CAD build for the part. Positions are in the model's coordinates, mm. Face numbers are marked on the shaded views. A direction names the side the tool comes from. Give positions to 0.01 mm unless a question says otherwise; leave off trailing zeros. Write each loop counter-clockwise with the first axis right and the second up, starting at its lowest first coordinate (ties: lowest second). Pieces come first, ordered by that corner, then holes. Notation, with made-up numbers: (85, -30.5) - (126, -30.5) arc R24 cw to (126, 5.5) - close; hole circle Ø10 at (74.5, 45). An arc over 180 degrees is marked (long way). Answer as a JSON object with one key per item and string values.
from build123d import *

# Parameters (mm, degrees)
BOSS_EXTRU_1_DEPTH           = 12
ESQUISSE10_R                 = 1.6
ENL_V_MAT_EXTRU_6_DEPTH      = 96.463780217
ENL_V_MAT_EXTRU_1_DEPTH      = 96.463780217
ENL_V_MAT_EXTRU_2_DEPTH      = 11
ESQUISSE4_W                  = 6
ESQUISSE4_H                  = 3
ENL_V_MAT_EXTRU_3_DEPTH      = 9.5
ESQUISSE11_R                 = 5.075
ENL_V_MAT_EXTRU_7_DEPTH      = 2
R_P_TITION_CIRCULAIRE1_COUNT = 3
CHANFREIN1_SIZE              = 0.5


with BuildPart() as part:
    # Esquisse1 → Boss.-Extru.1 (new body)
    with BuildSketch(Plane(origin=(0, 0, 0), x_dir=(1, 0, 0), z_dir=(0, 1, 0))):
        Polygon((-62, -35.79571669), (62, -35.79571669), (0, 71.59143338), align=None)
    extrude(amount=BOSS_EXTRU_1_DEPTH)

    # Esquisse10 → Enlèv. mat.-Extru.6 (cut, through all)
    with BuildSketch(Plane(origin=(0, 12, 0), x_dir=(1, 0, 0), z_dir=(0, 1, 0))):
        with Locations(Location((0, 54, 0), (0, 0, 270))):
            Circle(ESQUISSE10_R)
        with Locations(Location((46.765371804, -27, 0), (0, 0, 270))):
            Circle(ESQUISSE10_R)
        with Locations(Location((-46.765371804, -27, 0), (0, 0, 270))):
            Circle(ESQUISSE10_R)
    extrude(amount=-ENL_V_MAT_EXTRU_6_DEPTH, mode=Mode.SUBTRACT)

    # Esquisse2 → Enlèv. mat.-Extru.1 (cut, through all)
    with BuildSketch(Plane(origin=(0, 12, 0), x_dir=(1, 0, 0), z_dir=(0, 1, 0))):
        Polygon((-8.660254038, 56.59143338), (8.660254038, 56.59143338), (0, 71.59143338), align=None)
        Polygon((62, -35.79571669), (53.339745962, -20.79571669), (44.679491924, -35.79571669), align=None)
        Polygon((-62, -35.79571669), (-44.679491924, -35.79571669), (-53.339745962, -20.79571669), align=None)
    extrude(amount=-ENL_V_MAT_EXTRU_1_DEPTH, mode=Mode.SUBTRACT)

    # Esquisse3 → Enlèv. mat.-Extru.2 (cut)
    with BuildSketch(Plane(origin=(0, 12, 0), x_dir=(1, 0, 0), z_dir=(0, 1, 0))):
        with BuildLine():
            Line((44.679491924, -11.79571669), (12.124355653, 44.59143338))
            ThreePointArc((12.124355653, 44.59143338), (0, 51.59143338), (-12.124355653, 44.59143338))
            Line((-12.124355653, 44.59143338), (-44.679491924, -11.79571669))
            ThreePointArc((-44.679491924, -11.79571669), (-44.679491924, -25.79571669), (-32.555136271, -32.79571669))
            Line((-32.555136271, -32.79571669), (32.555136271, -32.79571669))
            ThreePointArc((32.555136271, -32.79571669), (44.679491924, -25.79571669), (44.679491924, -11.79571669))
        make_face()
    extrude(amount=-ENL_V_MAT_EXTRU_2_DEPTH, mode=Mode.SUBTRACT)

    # Esquisse4 → Enlèv. mat.-Extru.3 (cut)
    with BuildSketch(Plane(origin=(0, 12, 0), x_dir=(1, 0, 0), z_dir=(0, 1, 0))):
        Polygon((29.901923789, 13.799782134), (26.901923789, 18.995934556), (29.5, 20.495934556), (32.5, 15.299782134), align=None)
        with Locations((0, -34.29571669)):
            Rectangle(ESQUISSE4_W, ESQUISSE4_H)
        Polygon((-29.5, 20.495934556), (-26.901923789, 18.995934556), (-29.901923789, 13.799782134), (-32.5, 15.299782134), align=None)
    extrude(amount=-ENL_V_MAT_EXTRU_3_DEPTH, mode=Mode.SUBTRACT)

    # Esquisse11 → Enlèv. mat.-Extru.7 (cut)
    with BuildSketch(Plane(origin=(0, 0, 32.79571669), x_dir=(-1, 0, 0), z_dir=(0, 0, -1))):
        with Locations((-17.555136271, 6.5)):
            Circle(ESQUISSE11_R)
        with Locations(Location((17.555136271, 6.5, 0), (0, 0, 180))):
            Circle(ESQUISSE11_R)
    enl_v_mat_extru_7 = extrude(amount=-ENL_V_MAT_EXTRU_7_DEPTH, mode=Mode.SUBTRACT)

    # Répétition circulaire1: Enlèv. mat.-Extru.7 ×3 about axis
    r_p_tition_circulaire1_axis = Axis((0, 0, 0), (0, 1, 0))
    for i in range(1, R_P_TITION_CIRCULAIRE1_COUNT):
        add(enl_v_mat_extru_7.rotate(r_p_tition_circulaire1_axis, i * 360 / R_P_TITION_CIRCULAIRE1_COUNT), mode=Mode.SUBTRACT)

    # Chanfrein1
    # the kernel refuses this chamfer: 0.5 mm, written as the material it takes off along each edge
    with BuildSketch(Plane(origin=(17.555136271, 6.5, 32.79571669), x_dir=(-1, 0, 0), z_dir=(0, -1, 0))) as chanfrein1_piece_1_section:
        Polygon((5.075 + CHANFREIN1_SIZE, 0), (5.075, -CHANFREIN1_SIZE), (5.075, 0), align=None)
    chanfrein1_piece_1 = revolve(axis=Axis((17.555136271, 6.5, 32.79571669), (0, 0, -1)), mode=Mode.PRIVATE)
    chanfrein1_piece_1 = split(chanfrein1_piece_1, bisect_by=Plane(origin=(22.868441697, 1, 33.034022115), z_dir=(0, 1, 0)), keep=Keep.TOP, mode=Mode.PRIVATE)
    add(chanfrein1_piece_1, mode=Mode.SUBTRACT)
    with BuildSketch(Plane(origin=(-17.555136271, 6.5, 32.79571669), x_dir=(1, 0, 0), z_dir=(0, 1, 0))) as chanfrein1_piece_2_section:
        Polygon((5.075 + CHANFREIN1_SIZE, 0), (5.075, -CHANFREIN1_SIZE), (5.075, 0), align=None)
    chanfrein1_piece_2 = revolve(axis=Axis((-17.555136271, 6.5, 32.79571669), (0, 0, -1)), mode=Mode.PRIVATE)
    chanfrein1_piece_2 = split(chanfrein1_piece_2, bisect_by=Plane(origin=(-22.868441724, 1, 33.034022142), z_dir=(0, 1, 0)), keep=Keep.TOP, mode=Mode.PRIVATE)
    add(chanfrein1_piece_2, mode=Mode.SUBTRACT)
    with BuildSketch(Plane(origin=(-19.624355653, 6.5, -31.601052323), x_dir=(-0.5000000000000007, 0, 0.8660254037844384), z_dir=(0, 1, 0))) as chanfrein1_piece_3_section:
        Polygon((5.075 + CHANFREIN1_SIZE, 0), (5.075, -CHANFREIN1_SIZE), (5.075, 0), align=None)
    chanfrein1_piece_3 = revolve(axis=Axis((-19.624355653, 6.5, -31.601052323), (0.8660254037844384, 0, 0.5000000000000004)), mode=Mode.PRIVATE)
    chanfrein1_piece_3 = split(chanfrein1_piece_3, bisect_by=Plane(origin=(-17.174081503, 1, -36.32166255), z_dir=(0, 1, 0)), keep=Keep.TOP, mode=Mode.PRIVATE)
    add(chanfrein1_piece_3, mode=Mode.SUBTRACT)
    with BuildSketch(Plane(origin=(-37.179491924, 6.5, -1.194664367), x_dir=(0.4999999999999994, 0, -0.866025403784439), z_dir=(0, -1, 0))) as chanfrein1_piece_4_section:
        Polygon((5.075 + CHANFREIN1_SIZE, 0), (5.075, -CHANFREIN1_SIZE), (5.075, 0), align=None)
    chanfrein1_piece_4 = revolve(axis=Axis((-37.179491924, 6.5, -1.194664367), (0.8660254037844384, 0, 0.5000000000000004)), mode=Mode.PRIVATE)
    chanfrein1_piece_4 = split(chanfrein1_piece_4, bisect_by=Plane(origin=(-40.04252319, 1, 3.287640397), z_dir=(0, 1, 0)), keep=Keep.TOP, mode=Mode.PRIVATE)
    add(chanfrein1_piece_4, mode=Mode.SUBTRACT)
    with BuildSketch(Plane(origin=(37.179491924, 6.5, -1.194664367), x_dir=(-0.4999999999999992, 0, -0.866025403784439), z_dir=(0, 1, 0))) as chanfrein1_piece_5_section:
        Polygon((5.075 + CHANFREIN1_SIZE, 0), (5.075, -CHANFREIN1_SIZE), (5.075, 0), align=None)
    chanfrein1_piece_5 = revolve(axis=Axis((37.179491924, 6.5, -1.194664367), (-0.8660254037844388, 0, 0.49999999999999983)), mode=Mode.PRIVATE)
    chanfrein1_piece_5 = split(chanfrein1_piece_5, bisect_by=Plane(origin=(40.042523227, 1, 3.287640407), z_dir=(0, 1, 0)), keep=Keep.TOP, mode=Mode.PRIVATE)
    add(chanfrein1_piece_5, mode=Mode.SUBTRACT)
    with BuildSketch(Plane(origin=(19.624355653, 6.5, -31.601052323), x_dir=(0.4999999999999997, 0, 0.8660254037844387), z_dir=(0, -1, 0))) as chanfrein1_piece_6_section:
        Polygon((5.075 + CHANFREIN1_SIZE, 0), (5.075, -CHANFREIN1_SIZE), (5.075, 0), align=None)
    chanfrein1_piece_6 = revolve(axis=Axis((19.624355653, 6.5, -31.601052323), (-0.8660254037844388, 0, 0.49999999999999983)), mode=Mode.PRIVATE)
    chanfrein1_piece_6 = split(chanfrein1_piece_6, bisect_by=Plane(origin=(17.174081493, 1, -36.321662513), z_dir=(0, 1, 0)), keep=Keep.TOP, mode=Mode.PRIVATE)
    add(chanfrein1_piece_6, mode=Mode.SUBTRACT)


solid = part.part
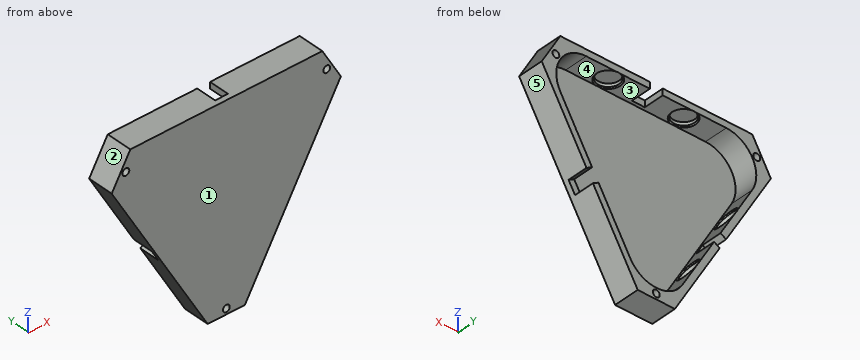
(1) Pull direction Z, two halves, no side cores. Call the marked faces 1, 2 and 3: pulls with the +Z half, pulls with the -Z half, needs draft (parallel to the pull), parting line crosses it, or undercut.
Answer key:
{"face 1": "needs draft", "face 2": "pulls with the +Z half", "face 3": "undercut"}
(2) Saw through at B-B, the plane z = -54. Give the cut face in (x, y), and give its area (3 significant figures).
Answer key:
{"outline": "(-10.16, 0) - (-1.6, 0) - (-1.6, 12) - (-10.16, 12) - close; (1.6, 0) - (10.16, 0) - (10.16, 12) - (1.6, 12) - close", "area": "205 mm²"}
(3) Probe L1, parallel to X at y = 3, z = 27; L2, parallel to Y at x = -22, z = 22; L3, parallel to Z at x = 14.5, y = 3.5. List the from-to ranges inside material, lowest first. Write a range as [from, to].
Answer key:
{"L1": "x = [-49.76, -48.37], [-45.17, -43.9], [43.9, 45.17], [48.37, 49.76]", "L2": "y = [0, 1]", "L3": "z = [-46.48, -40.48], [34.8, 35.8]"}
(4) 3-axis set-ups, long thin cutter, end or side, ignore diameter. For the marked faces 4 and 5: which of +Z, -Z, +X, -X, +Y, -Y reach the whole face in a straight line?
Answer key:
{"face 4": "+Y", "face 5": "-Z, +X, +Y, -Y"}
(5) Saw through at A-A, the plane x = 0. Give the cut face in (y, z).
Answer key:
{"outline": "(0, -56.59) - (12, -56.59) - (12, -55.6) - (0, -55.6) - close; (0, -52.4) - (12, -52.4) - (12, -51.59) - (1, -51.59) - (1, 32.8) - (2.5, 32.8) - (2.5, 35.8) - (0, 35.8) - close"}
(6) Saw through at D-D, the plane z = 27. Give the cut face in (x, y), and give its area (3 significant figures).
Answer key:
{"outline": "(-49.76, 0) - (-48.37, 0) - (-48.37, 12) - (-49.76, 12) - close; (-45.17, 0) - (45.17, 0) - (45.17, 12) - (43.9, 12) - (43.9, 1) - (-43.9, 1) - (-43.9, 12) - (-45.17, 12) - close; (48.37, 0) - (49.76, 0) - (49.76, 12) - (48.37, 12) - close", "area": "152 mm²"}
(7) Saw through at C-C, the plane y = 6.5. State how many separate pieces and enclosed holes the cut face has, and give its area (3 significant figures).
Answer key:
{"separate pieces": "3", "enclosed holes": "3", "area": "881 mm²"}
(8) Flat gauge pins, fed straight in: P1, Ø3, axis at y = 10, z = -0.5, coming from the +X side; P2, Ø0.9, axis at y = 8, z = 33.5, coming from the -X side; P3, Ø1.5, axis at y = 1.5, z = -1.5, coming from the -X side. Where does each tip first touch, or does it go through?
Answer key:
{"P1": "stops at x = 41.91", "P2": "stops at x = -46.26", "P3": "stops at x = -40.9"}
